from build123d import *

# Parameters (mm, degrees)
F0_R            = 59.5854737817
F0_R_2          = 5
F1_DEPTH        = 25
F3_D            = 10
F3_DEPTH        = 35
F3_TIP          = 3.0043030951
F3_COPIES_COUNT = 6


# Not quite as in the source:
# - a pattern or mirror of a feature is missing from the dataset's text; its kind, count and spacing are read off the source's solid


with BuildPart() as f1:
    # F0 (on Front) → F1 (new body)
    with BuildSketch(Plane.XZ):
        Circle(F0_R)
        with BuildLine():
            Line((-9.7349431967, -36.997402159), (-9.7675768508, -30.9974909059))
            ThreePointArc((-9.7675768508, -30.9974909059), (-0.1743718668, 32.499532219), (10.099630663, -30.8908960775))
            Line((10.099630663, -30.8908960775), (10.2647609802, -36.8886233119))
            Line((10.2647609802, -36.8886233119), (-9.7349431967, -36.997402159))
        make_face(mode=Mode.SUBTRACT)
        with Locations((0, 45)):
            Circle(F0_R_2, mode=Mode.SUBTRACT)
        with Locations((0, 45)):
            Circle(F0_R_2)
    extrude(amount=F1_DEPTH)

    # F3
    with Locations(Plane.XZ.offset(25)):
        with Locations((0, 45)):
            f3 = Hole(F3_D / 2, depth=F3_DEPTH)
            with Locations((0, 0, -(F3_DEPTH + F3_TIP / 2))):  # 118° drill point
                Cone(0, F3_D / 2, F3_TIP, mode=Mode.SUBTRACT)

    # F3_copies: F3 ×6 about axis
    f3_copies_axis = Axis((0, 0, 0), (0, 1, 0))
    for i in range(1, F3_COPIES_COUNT):
        add(f3.rotate(f3_copies_axis, i * 360 / F3_COPIES_COUNT), mode=Mode.SUBTRACT)


solid = f1.part
Build history of the part. All positions in model axes, mm. Round coordinates to 2 decimals unless told otherwise and drop trailing zeros. Loops run counter-clockwise (first coordinate to the right, second up) from the corner with the lowest first, then second, coordinate; pieces in that order, holes last. Notation, with made-up numbers: (-8, -16.5) -> (16, -16.5) arc R16 ccw to (16, -8.5) -> close; hole circle Ø1 at (-0.5, 41.5). An arc over 180 degrees is marked (long way). Use CSV: the item, a comma, the result in double quotes. Start each with the question number.
Q1. Mould opens along X. For faces 1 (the face through (-33.976, -12.325, -22.28)), 2 (the face through (-43.92, -12.32, 40.27)), 3 (the face through (26, 0, -26)), 4 (the face through (35.286, -12.325, 19.121)) say: +X half, -X half, draft (parallel to the pull), parting line (faces both ways), or undercut.
Q2. Saw through at C-C on y = -21.5. Give the cut face in (x, z), and give its area (3 significant figures).
Q3. Flat gauge pins, fed straight in: pin 1 Ø16 at (x, z) = (0, 45) entering from +Y; pin 2 Ø6 at (y, z) = (-5, 17.5) entering from +X; pin 3 Ø3 at (y, z) = (-12, 9) entering from +X; pin 4 Ø12 at (y, z) = (-21.5, 16) entering from +X. Where does each tip first touch, or does it go through?
Q4. Saw through at A-A on z = 0. Give the cut face in (x, y).
Q5. Saw through at B-B on x = -29. Give the cut face in (y, z).
Q6. Saw through at D-D on x = 0. Give the cut face in (y, z), and give its area (3 significant figures).
Q7. Drill centre lines: L1, parallel to X at y = -7, z = -20.5; L2, parallel to Z at x = -43.5, y = -3; L3, parallel to X at y = -11.5, z = -18. Where is each one in solid material? Low to high.
Solutions:
1,face 1,"undercut"
1,face 2,"parting line"
1,face 3,"draft"
1,face 4,"undercut"
2,outline,"circle Ø119.17 at (0, 0); hole circle Ø10 at (-38.97, -22.5); hole circle Ø10 at (-38.97, 22.5); hole (-9.77, -31) -> (-9.73, -37) -> (10.26, -36.89) -> (10.1, -30.89) arc R32.5 ccw (long way) to start; hole circle Ø10 at (0, -45); hole circle Ø10 at (0, 45); hole circle Ø10 at (38.97, -22.5); hole circle Ø10 at (38.97, 22.5)"
2,area,"7,270 mm^2"
3,pin 1,"stops at y = 0"
3,pin 2,"stops at x = 57.79"
3,pin 3,"stops at x = 59.11"
3,pin 4,"stops at x = 58.74"
4,outline,"(-59.59, -25) -> (-32.5, -25) -> (-32.5, 0) -> (-59.59, 0) -> close; (32.5, -25) -> (59.59, -25) -> (59.59, 0) -> (32.5, 0) -> close"
5,outline,"(-25, -52.05) -> (0, -52.05) -> (0, -14.67) -> (-25, -14.67) -> close; (-25, 14.67) -> (0, 14.67) -> (0, 52.05) -> (-25, 52.05) -> close"
6,outline,"(-25, -59.59) -> (0, -59.59) -> (0, -50) -> (-25, -50) -> close; (-25, -40) -> (0, -40) -> (0, -36.94) -> (-25, -36.94) -> close; (-25, 32.5) -> (0, 32.5) -> (0, 40) -> (-25, 40) -> close; (-25, 50) -> (0, 50) -> (0, 59.59) -> (-25, 59.59) -> close"
6,area,"743 mm^2"
7,L1,"x = -55.95 to -43.55, -34.39 to -25.22, 25.22 to 34.39, 43.55 to 55.95"
7,L2,"z = -40.72 to -24.62, -20.38 to 20.38, 24.62 to 40.72"
7,L3,"x = -56.8 to -41.15, -36.79 to -27.06, 27.06 to 36.79, 41.15 to 56.8"
